Here's how the part is built. I have some questions about the finished solid (model axes, mm). A direction names the side the tool comes from. Round coordinates to 2 decimals unless told otherwise and drop trailing zeros. Loops run counter-clockwise (first coordinate to the right, second up) from the corner with the lowest first, then second, coordinate; pieces in that order, holes last. Notation, with made-up numbers: M 55.5,5 L 66.5,5 A11 cw 66.5,23 Z; hole C -18.5,-23.75 d2. An arc over 180 degrees is marked long. Write each question's results on one line, items separated by ' | '. Start each with the question number.
```python
from build123d import *

# Parameters (mm, degrees)
SKETCH_1_W           = 15
SKETCH_1_H           = 2.54
EXTRUDE_1_DEPTH      = 2.5
EXTRUDE_2_DEPTH      = 7
EXTRUDE_2_DEPTH_BACK = 5
SKETCH_2_W           = 1
SKETCH_2_H           = 1


with BuildPart() as part:
    # Эскиз1 → Бобышка-Вытянуть1 (new body)
    with BuildSketch(Plane.XY):
        Rectangle(SKETCH_1_W, SKETCH_1_H)
    extrude(amount=EXTRUDE_1_DEPTH)

    # Эскиз2 → Бобышка-Вытянуть2 (add, two sides: drawn at the far end of the back side and taken through both)
    with BuildSketch(Plane(origin=(0, 0, 0), x_dir=(-1, 0, 0), z_dir=(0, 0, -1)).offset(-EXTRUDE_2_DEPTH_BACK)):
        with Locations((-3.75, 0)):
            Rectangle(SKETCH_2_W, SKETCH_2_H)
        with Locations((-6.25, 0)):
            Rectangle(SKETCH_2_W, SKETCH_2_H)
        with Locations((-1.25, 0)):
            Rectangle(SKETCH_2_W, SKETCH_2_H)
        with Locations((1.25, 0)):
            Rectangle(SKETCH_2_W, SKETCH_2_H)
        with Locations((3.75, 0)):
            Rectangle(SKETCH_2_W, SKETCH_2_H)
        with Locations((6.25, 0)):
            Rectangle(SKETCH_2_W, SKETCH_2_H)
    extrude(amount=EXTRUDE_2_DEPTH + EXTRUDE_2_DEPTH_BACK)


solid = part.part
```
Item 1: I'm going to push flat-ended pins straight in: pin 1 (1.1 mm diameter, centred on x = -6.5, z = -2, fed in from +Y); pin 2 (0.8 mm diameter, centred on x = 1.5, z = -4.5, fed in from -Y); pin 3 (5 mm diameter, centred on x = 1.5, z = -2, fed in from -Y); pin 4 (0.8 mm diameter, centred on y = 0, z = -4.5, fed in from -X). Where does each tip first touch, or does it pass through?
Item 2: If we mould it in two halves opening along X, with no side actions, what happens to faces 6 (the face through (-4.25, 0, 4)), 7 (the face through (1, 0, 5)), 8 (the face through (-6.75, 0, 4))? For each: released by +X, released by -X, zero draft, split by the parting line, or undercut.
Item 3: If we section it at B-B on x = 3.5: Please give me the cut outline in (y, z), and give its area (4 significant figures).
Item 4: Which directions (+Z, -Z, +X, -X, +Y, -Y) give clear straight access to the entire face, cutting with the end or side of a thin tool? Please do faces 1 (the face through (6, -0.5, 4)), 2 (the face through (-1, 0.5, -3)), 3 (the face through (3.25, 0, -3)), 4 (the face through (-4, -0.5, -3)), 5 (the face through (5.75, 0, 4)).
Item 5: If we section it at C-C on y = 0.75: Please give me the cut outline in (x, z), and give its area (3 significant figures).
Item 6: If we section it at A-A on z = -1: Please give me the cut outline in (x, y), and give its area (3 significant figures).
Item 7: If we section it at D-D on x = 5.5: Please give me the cut outline in (y, z), and give its area (3 significant figures).
Item 8: I need wall thicknesses on L1, parallel to X at y = 0.1, z = -0.75; L2, parallel to Z at x = 0.25, y = 1.1; L3, parallel to Y at x = 1.5, z = -2.5. Which ranges of each line are inside material? Lowest first, please.
Numbers:
1) pin 1: y = 0.5 | pin 2: y = -0.5 | pin 3: y = -1.27 | pin 4: x = -6.75
2) face 6: undercut | face 7: zero draft | face 8: released by -X
3) outline: M -1.27,0 L -0.5,0 L -0.5,-7 L 0.5,-7 L 0.5,0 L 1.27,0 L 1.27,2.5 L 0.5,2.5 L 0.5,5 L -0.5,5 L -0.5,2.5 L -1.27,2.5 Z | area: 15.85 mm²
4) face 1: +Z, +X, -X, -Y | face 2: -Z, +X, -X, +Y | face 3: -Z, +Y, -Y | face 4: -Z, +X, -X, -Y | face 5: +Z, +Y, -Y
5) outline: M -7.5,0 L 7.5,0 L 7.5,2.5 L -7.5,2.5 Z | area: 37.5 mm²
6) outline: M -6.75,-0.5 L -5.75,-0.5 L -5.75,0.5 L -6.75,0.5 Z; M -4.25,-0.5 L -3.25,-0.5 L -3.25,0.5 L -4.25,0.5 Z; M -1.75,-0.5 L -0.75,-0.5 L -0.75,0.5 L -1.75,0.5 Z; M 0.75,-0.5 L 1.75,-0.5 L 1.75,0.5 L 0.75,0.5 Z; M 3.25,-0.5 L 4.25,-0.5 L 4.25,0.5 L 3.25,0.5 Z; M 5.75,-0.5 L 6.75,-0.5 L 6.75,0.5 L 5.75,0.5 Z | area: 6.00 mm²
7) outline: M -1.27,0 L 1.27,0 L 1.27,2.5 L -1.27,2.5 Z | area: 6.35 mm²
8) L1: -6.75 to -5.75, -4.25 to -3.25, -1.75 to -0.75, 0.75 to 1.75, 3.25 to 4.25, 5.75 to 6.75 | L2: 0 to 2.5 | L3: -0.5 to 0.5
